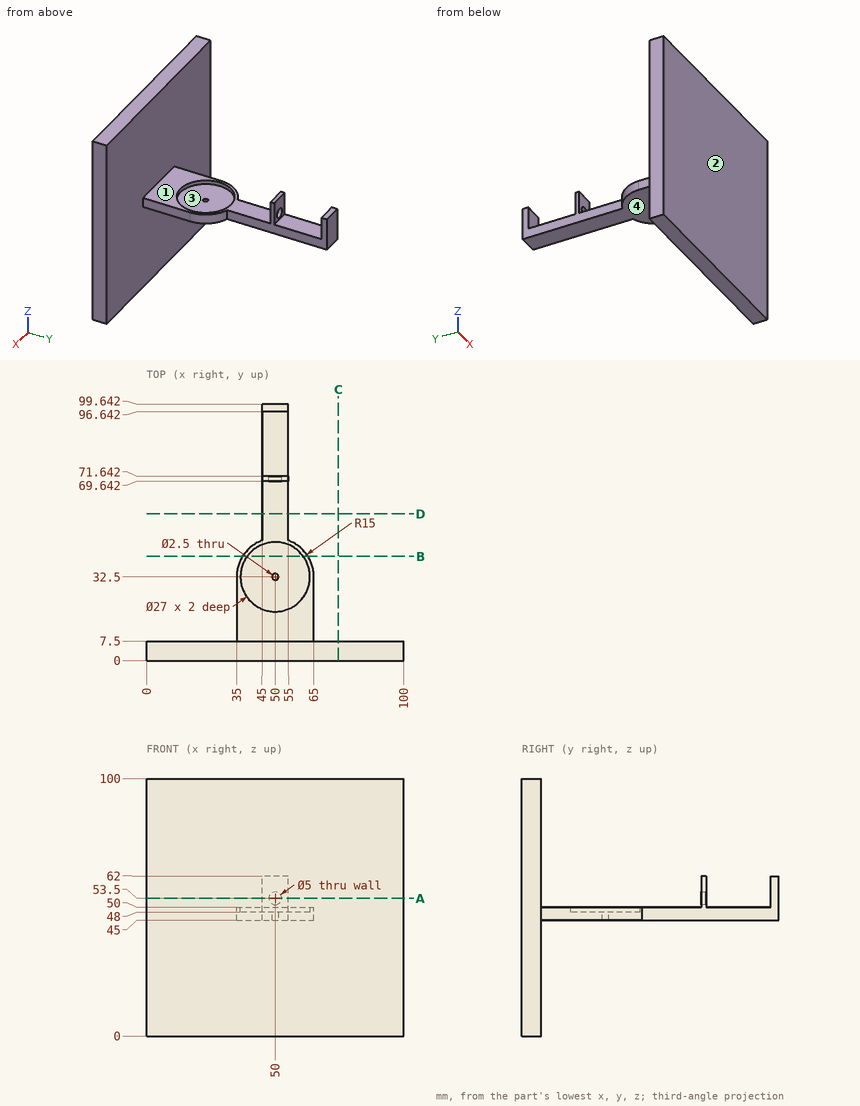
Print and shaded views of the part. All mm, measured from the part's lowest x, y and z. Coordinates: 2 decimals unless noted, no trailing zeros. Write each loop counter-clockwise with the first axis right and the second up, starting at its lowest first coordinate (ties: lowest second). Pieces come first, ordered by that corner, then holes.
(1) Two-plate mould, pull along Y, no slides. Class the marked faces 1, 2, 3 and 4: +Y half, -Y half, draft (parallel to the pull), parting line (faces both ways), or undercut.
(2) Cut at D-D, the plane y = 57. List the corners of the cut face in (x, z).
(3) Cut at B-B, the plane y = 40.5. List the corners of the cut face in (x, z).
(4) Cut at C-C, the plane x = 74.5. List the corners of the cut face in (y, z), and give its area (3 significant figures).
(5) Cut at A-A, the plane z = 53.5. List the corners of the cut face in (x, y), and give its area (3 significant figures).
(6) Flat gauge pins, fed straight in: pin 1 (1 mm diameter, centred on x = 50, y = 71, fed in from +Z); pin 2 (8.5 mm diameter, centred on y = 78, z = 51.5, fed in from +X); pin 3 (2.5 mm diameter, centred on y = 19, z = 46.5, fed in from +X). Where does each tip first touch, or does it go through?
(7) Drill centre lines: probe 1 along Y at (x, z) = (50, 48.75); probe 2 along Y at (x, z) = (50, 45.6); probe 3 along Z at (x, y) = (39.5, 32). Where is each one in solid material? Low to high.
Geometry says:
1. face 1: undercut
1. face 2: -Y half
1. face 3: undercut
1. face 4: draft
2. outline: (45, 45) - (55, 45) - (55, 50) - (45, 50) - close
3. outline: (37.31, 45) - (62.69, 45) - (62.69, 50) - (60.87, 50) - (60.87, 48) - (39.13, 48) - (39.13, 50) - (37.31, 50) - close
4. outline: (0, 0) - (7.5, 0) - (7.5, 100) - (0, 100) - close
4. area: 750 mm2
5. outline: (0, 0) - (100, 0) - (100, 7.5) - (0, 7.5) - close; (45, 69.64) - (47.5, 69.64) - (47.5, 71.64) - (45, 71.64) - close; (45, 96.64) - (55, 96.64) - (55, 99.64) - (45, 99.64) - close; (52.5, 69.64) - (55, 69.64) - (55, 71.64) - (52.5, 71.64) - close
5. area: 790 mm2
6. pin 1: stops at z = 62
6. pin 2: stops at x = 55
6. pin 3: stops at x = 65
7. probe 1: y = 0 to 19, 46 to 99.64
7. probe 2: y = 0 to 31.25, 33.75 to 99.64
7. probe 3: z = 45 to 48
